Source: three-view drawing plus pictorial views. Frame: mm from the lowest corner of the part. A direction names the side the tool comes from. Give positions to 0.01 mm unless a question says otherwise; leave off trailing zeros. Order: outer loops, then holes, each group sorted by start corner. A loop starts at its lowest first (then second) coordinate and runs counter-clockwise, first axis right, second up. Notation, with made-up numbers: (-22, 38.5) -> (32, 38.5) arc R37 ccw to (32, 77.5) -> close; hole circle Ø7 at (3.25, 38). An arc over 180 degrees is marked (long way). One line per question, with ' | ' between items.
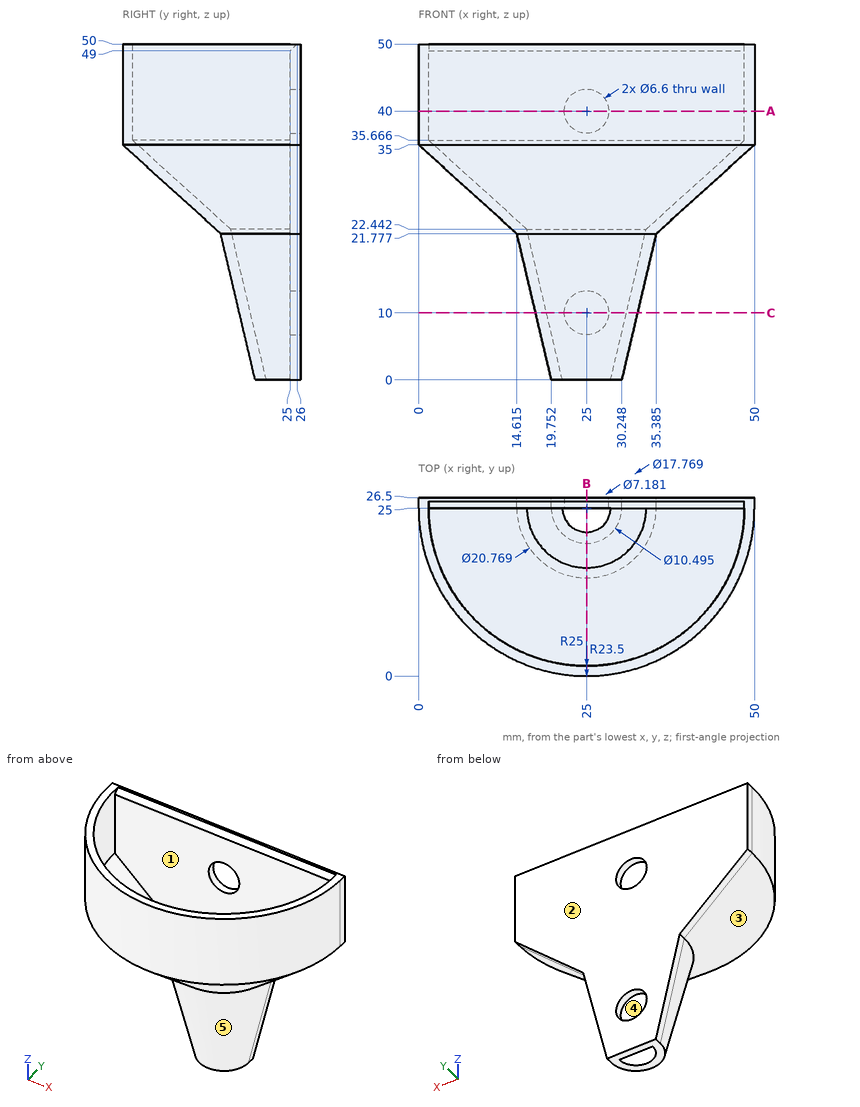
1) Contact query for flat-ended pins moving along their axis: pin 1 Ø2 at (y, z) = (17, 16) entering from -X (1 decimal); pin 2 Ø7.5 at (x, z) = (25, 10) entering from +Y; pin 3 Ø5 at (x, y) = (40, 17) entering from -Z; pin 4 Ø8 at (y, z) = (18, 44.5) entering from +X. Output: stop coordinate, or through.
Check result:
pin 1: stops at x = 19.3 | pin 2: stops at y = 26.5 | pin 3: stops at z = 25.5 | pin 4: stops at x = 49.82
2) Set-up query: the marked faces 4 and 5. Return all of +Z, -Z, +X, -X, +Y, -Y with unobstructed straight access to the full face (end or side cutting, diameter ignored); none if empty.
Check result:
face 4: +Z | face 5: -Z, -Y
3) Section A-A on z = 40. Return loops of the section in (x, y).
Check result:
outline: (0, 25) arc R25 ccw to (50, 25) -> (50, 26.5) -> (28.3, 26.5) -> (28.3, 25) -> (48.5, 25) arc R23.5 cw to (1.5, 25) -> (21.7, 25) -> (21.7, 26.5) -> (0, 26.5) -> close
4) Pull-direction query (X, two-part tool) for the marked faces 1, 2 and 3; classes: +X half, -X half, draft (parallel to the pull), parting line (faces both ways), or undercut.
Check result:
face 1: undercut | face 2: draft | face 3: parting line
5) Section B-B on x = 25. Return loops of the section in (y, z) (1 decimal).
Check result:
outline: (0, 35) -> (14.6, 21.8) -> (19.8, 0) -> (21.4, 0) -> (16.1, 22.4) -> (1.5, 35.7) -> (1.5, 50) -> (0, 50) -> close; (25, 0) -> (26.5, 0) -> (26.5, 6.7) -> (25, 6.7) -> close; (25, 13.3) -> (26.5, 13.3) -> (26.5, 36.7) -> (25, 36.7) -> close; (25, 43.3) -> (26.5, 43.3) -> (26.5, 50) -> (26, 50) -> (25, 49) -> close
6) Section C-C on z = 10. Return loops of the section in (x, y).
Check result:
outline: (17.39, 25) arc R7.61 ccw to (32.61, 25) -> (32.61, 26.5) -> (28.3, 26.5) -> (28.3, 25) -> (30.95, 25) arc R5.95 cw to (19.05, 25) -> (21.7, 25) -> (21.7, 26.5) -> (17.39, 26.5) -> close
7) Material intervals for probe 1 along Z at (x, y) = (25, 26.1); probe 2 along Z at (x, y) = (25, 25.8); probe 3 along Y at (x, z) = (25.5, 30) (1 decimal), sorted ascending. Write a range as from..to.
Check result:
probe 1: z = 0..6.7, 13.3..36.7, 43.3..50 | probe 2: z = 0..6.7, 13.3..36.7, 43.3..49.8 | probe 3: y = 5.5..7.8, 25..26.5
